Can you work these out from the model? Positions are in its coordinate system, mm. A direction names the side the tool comes from. Give positions to 0.01 mm unless a question says otherwise; leave off trailing zeros. Loops run counter-clockwise (first coordinate to the right, second up) from the corner with the lowest first, then second, coordinate; pieces in that order, holes last. Notation, with made-up numbers: (44, 27) - (51, 27) arc R20 ccw to (51, 42) - close; hole circle Ø11 at (-15.75, 10.5). An arc over 180 degrees is marked (long way). Write item = value, one per line.
from build123d import *

# Parameters (mm, degrees)
EXTRUDE_1_DEPTH = 8
EXTRUDE_2_DEPTH = 8


with BuildPart() as part:
    # Эскиз1 → Повернуть1 (revolve)
    with BuildSketch(Plane.XY, mode=Mode.PRIVATE) as revolve_1_sk:
        Polygon((0, 0), (-25, 0), (-25, 10), (-18, 17), (-12, 17), (-12, 20), (-5, 20), (-5, 28), (-5, 126.4), (-3.4, 128), (0, 128), align=None)
    revolve(revolve_1_sk.sketch.rotate(Axis((0, 0, 0), (0, 1, 0)), 180), axis=Axis((0, 0, 0), (0, 1, 0)))  # turned: the seam where the file's is

    # Эскиз2 → Бобышка-Вытянуть1 (add)
    with BuildSketch(Plane(origin=(0, 20, 0), x_dir=(1, 0, 0), z_dir=(0, 1, 0))):
        Polygon((0, 9.814954576), (-8.5, 4.907477288), (-8.5, -4.907477288), (0, -9.814954576), (8.5, -4.907477288), (8.5, 4.907477288), align=None)
    extrude(amount=EXTRUDE_1_DEPTH)

    # Эскиз3 → Бобышка-Вытянуть2 (add)
    with BuildSketch(Plane(origin=(0, 77.2, 0), x_dir=(1, 0, 0), z_dir=(0, 1, 0))):
        Polygon((8.5, 4.907477288), (0, 9.814954576), (-8.5, 4.907477288), (-8.5, -4.907477288), (0, -9.814954576), (8.5, -4.907477288), align=None)
    extrude(amount=EXTRUDE_2_DEPTH)

    # Эскиз4 → Вырез-Повернуть2 (revolve, cut)
    with BuildSketch(Plane.XY, mode=Mode.PRIVATE) as cut_revolve_2_sk:
        Polygon((-15.42820323, 85.2), (-8.5, 85.2), (-15.42820323, 81.2), align=None)
        Polygon((-15.42820323, 77.2), (-15.42820323, 81.2), (-8.5, 77.2), align=None)
        Polygon((-15.42820323, 28), (-15.42820323, 24), (-8.5, 28), align=None)
        Polygon((-15.42820323, 24), (-15.42820323, 20), (-8.5, 20), align=None)
    revolve(cut_revolve_2_sk.sketch.rotate(Axis((0, 128, 0), (0, -1, 0)), 180), axis=Axis((0, 128, 0), (0, -1, 0)), mode=Mode.SUBTRACT)  # turned: the seam where the file's is


solid = part.part
Q1. Which directions (+Z, -Z, +X, -X, +Y, -Y) give clear straight access to the entire face, cutting with the end or side of a thin tool? Please do faces 1 (the flat face through (5, 20, -8)), 2 (the conical face through (0.02, 27.82, 8.81)), 3 (the flat face through (-4.31, 81.144, 7.327)).
Output:
face_1 = none
face_2 = +Z
face_3 = +Z, -X, +Y
Q2. Imagine slicing it at A-A, the plane y = 61. Write out the boundary of the cut face in (x, z), then the cut area to 3 significant figures.
Output:
outline = circle Ø10 at (0, 0)
area = 78.5 mm2
Q3. I need wall thicknesses on L1, parallel to Y at x = -11.5, z = -6.5; L2, parallel to Y at x = 5.5, z = 10.5; L3, parallel to Z at x = 1, y = 52.5. Which ranges of each line are inside material? Lowest first, please.
Output:
L1 = 0 to 17
L2 = 0 to 20
L3 = -4.9 to 4.9
Q4. For pin 1 (4 mm diameter, centred on y = 86, z = 0.5, fed in from -X); pin 2 (3 mm diameter, centred on x = -4.5, z = 15, fed in from +Y); pin 3 (1 mm diameter, centred on x = -9, z = 16.5, fed in from +Y), each with a flat end and sliding along its axis, tell me the tip position at first contact or that it passes through.
Output:
pin_1 = -8.5
pin_2 = 17
pin_3 = 16.71
